Here's the drawing with two shaded views (mm, measured from the low corner). I have some questions. A direction names the side the tool comes from. Round coordinates to 2 decimals unless told otherwise and drop trailing zeros. Write each loop counter-clockwise with the first axis right and the second up, starting at its lowest first coordinate (ties: lowest second). Pieces come first, ordered by that corner, then holes. Notation, with made-up numbers: (-19, -24) -> (11, -24) arc R19 ccw to (11, -13) -> close; hole circle Ø7 at (-25, 27). An arc over 180 degrees is marked (long way). Use CSV: the item, a comma, the result in double quotes.
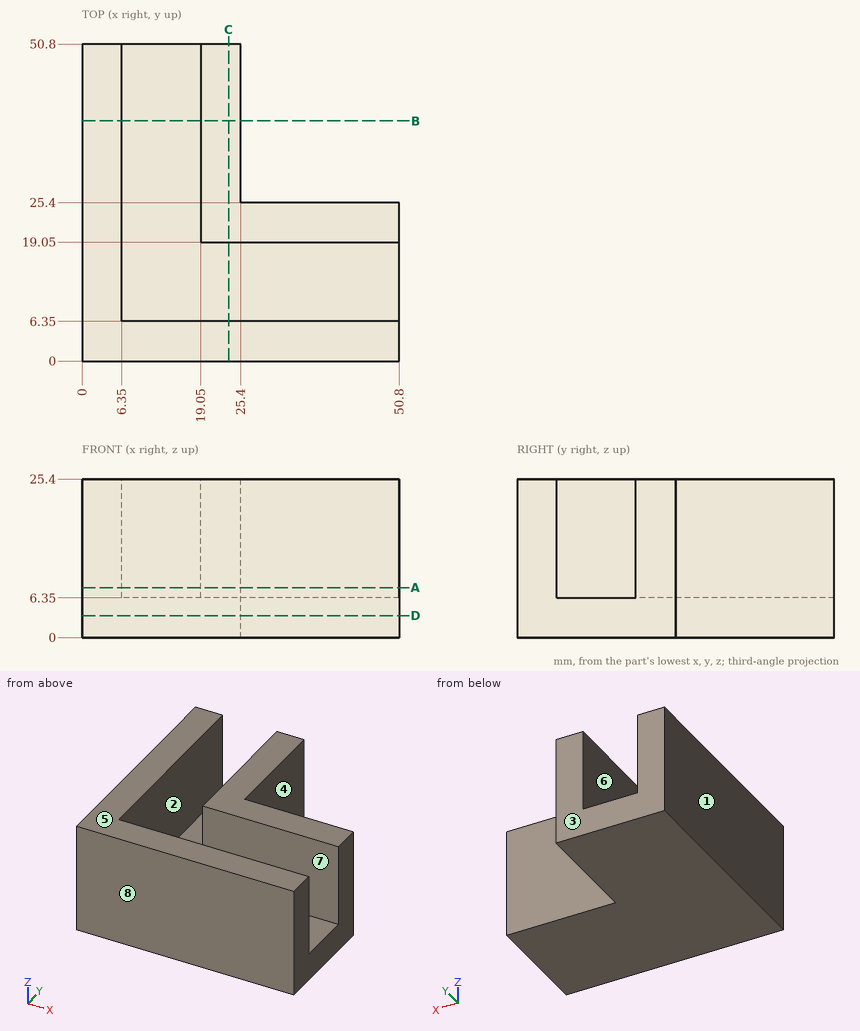
Q1. Suppose I cut it at C-C (x = 23.5). Write out the boundary of the cut face in (y, z).
Resolved:
outline,"(0, 0) -> (50.8, 0) -> (50.8, 25.4) -> (19.05, 25.4) -> (19.05, 6.35) -> (6.35, 6.35) -> (6.35, 25.4) -> (0, 25.4) -> close"
Q2. On a 3-axis mill with a long thin cutter (end or side, diameter ignored), from which of +Z, -Z, +X, -X, +Y, -Y can I reach the whole of each face in a straight line? I mean the marked faces 4, 5, 6, 7 and 8. Say none if no direction works.
Resolved:
face 4,"+Z, -Z, +X, +Y"
face 5,"+Z, +X, -X, +Y, -Y"
face 6,"+Z, +Y"
face 7,"+Z, +X"
face 8,"+Z, -Z, +X, -X, -Y"
Q3. Suppose I cut it at D-D (z = 3.5). Write out the boundary of the cut face in (x, y).
Resolved:
outline,"(0, 0) -> (50.8, 0) -> (50.8, 25.4) -> (25.4, 25.4) -> (25.4, 50.8) -> (0, 50.8) -> close"
Q4. Suppose I cut it at B-B (y = 38.5). Write out the boundary of the cut face in (x, z), and give its area (3 significant figures).
Resolved:
outline,"(0, 0) -> (25.4, 0) -> (25.4, 25.4) -> (19.05, 25.4) -> (19.05, 6.35) -> (6.35, 6.35) -> (6.35, 25.4) -> (0, 25.4) -> close"
area,"403 mm^2"
Q5. Please list where these lines run through material, in increasing order: probe 1 along X at (y, z) = (25, 17.5); probe 2 along X at (y, z) = (35, 20.75).
Resolved:
probe 1,"x = 0 to 6.35, 19.05 to 50.8"
probe 2,"x = 0 to 6.35, 19.05 to 25.4"
Q6. Suppose I cut it at A-A (z = 8). Write out the boundary of the cut face in (x, y).
Resolved:
outline,"(0, 0) -> (50.8, 0) -> (50.8, 6.35) -> (6.35, 6.35) -> (6.35, 50.8) -> (0, 50.8) -> close; (19.05, 19.05) -> (50.8, 19.05) -> (50.8, 25.4) -> (25.4, 25.4) -> (25.4, 50.8) -> (19.05, 50.8) -> close"
Q7. If we mould it in two halves opening along X, with no side actions, what happens to the marked faces 1, 2 and 3? For each: released by +X, released by -X, zero draft, split by the parting line, or undercut.
Resolved:
face 1,"released by -X"
face 2,"undercut"
face 3,"zero draft"
Q8. Will these pins go through, and if not, where does the flat tip stop? P1, Ø7.5, axis at y = 37.5, z = 18, coming from the +X side; P2, Ø1, axis at x = 33.5, z = 15.5, coming from the +Y side; P3, Ø5, axis at y = 12, z = 19.5, coming from the +X side.
Resolved:
P1,"stops at x = 25.4"
P2,"stops at y = 25.4"
P3,"stops at x = 6.35"
